from build123d import *

# Parameters (mm, degrees)
F0_W     = 122.6633450469
F0_H     = 164.7901384103
F0_W_2   = 102.3433450469
F0_H_2   = 144.4701384103
F1_DEPTH = 72.898
F2_R     = 8.301996535
F3_DEPTH = 244.094
F4_W     = 10.16
F4_H     = 88.5901384103
F5_DEPTH = 29.718


with BuildPart() as f1:
    # F0 (on Top) → F1 (new body)
    with BuildSketch(Plane.XY):
        with Locations((-22.7750174733, 0)):
            Rectangle(F0_W, F0_H)
        with Locations((-22.7750174733, 0)):
            Rectangle(F0_W_2, F0_H_2, mode=Mode.SUBTRACT)
    extrude(amount=F1_DEPTH)

    # F2 (on face) → F3 (cut)
    with BuildSketch(Plane(origin=(0, 82.3950692052, 0), x_dir=(-1, 0, 0), z_dir=(0, 1, 0))):
        with Locations((22.7750174733, 36.449)):
            Circle(F2_R)
    extrude(amount=-F3_DEPTH, mode=Mode.SUBTRACT)

    # F4 (on face) → F5 (cut)
    with BuildSketch(Plane.XY.offset(72.898)):
        with Locations((33.4766550502, 0)):
            Rectangle(F4_W, F4_H)
        with Locations((-79.0266899967, 0)):
            Rectangle(F4_W, F4_H)
    extrude(amount=-F5_DEPTH, mode=Mode.SUBTRACT)


solid = f1.part
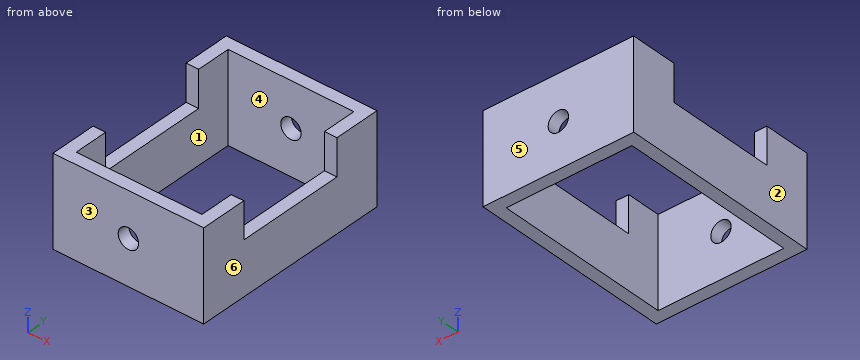
Input: part model. Units: mm. Frame: model coordinates. Face numbers are marked on the shaded views. A direction names the side the tool comes from. Coordinates: 2 decimals unless noted, no trailing zeros. Loops run counter-clockwise (first coordinate to the right, second up) from the corner with the lowest first, then second, coordinate; pieces in that order, holes last.
(1) Section D-D on z = 24.5. Return the cut outline in (x, y), then the cut area to 3 significant figures.
(2) Section B-B on x = 8. Return the cut outline in (y, z), then the cut area to 3 significant figures.
(3) Set-up query: the marked faces 1 and 2. Return all of +Z, -Z, +X, -X, +Y, -Y with unobstructed straight access to the full face (end or side cutting, diameter ignored); none if empty.
(4) Material intervals for probe 1 along X at (y, z) = (19, 43); probe 2 along Y at (x, z) = (-29.5, 24), sorted ascending.
(5) Section A-A on z = 54. Return the cut outline in (x, y), then the cut area to 3 significant figures.
(6) First-contact query: pin 1 Ø5 at (x, y) = (33.5, -4) entering from +Z; pin 2 Ø21.5 at (x, z) = (-22.78, 36.45) entering from -Y. Flat tips, straight axial feed; report the tip coordinate or a pass-through.
(7) Section C-C on y = -20. Return the cut outline in (x, z).
(8) Pull-direction query (Y, two-part tool) for the marked faces 3, 4, 5 and 6; classes: released by +Y, released by -Y, zero draft, split by the parting line, or undercut.
Data:
1. outline: (-84.11, -82.4) - (38.56, -82.4) - (38.56, 82.4) - (-84.11, 82.4) - close; hole (-73.95, -72.24) - (28.4, -72.24) - (28.4, 72.24) - (-73.95, 72.24) - close
1. area: 5,430 mm2
2. outline: (-82.4, 0) - (-72.24, 0) - (-72.24, 72.9) - (-82.4, 72.9) - close; (72.24, 0) - (82.4, 0) - (82.4, 72.9) - (72.24, 72.9) - close
2. area: 1,480 mm2
3. face 1: +Z, -Z
3. face 2: +Z, -Z, -X, +Y, -Y
4. probe 1: x = -84.11 to -73.95, 28.4 to 38.56
4. probe 2: y = -82.4 to -72.24, 72.24 to 82.4
5. outline: (-84.11, -82.4) - (38.56, -82.4) - (38.56, -44.3) - (28.4, -44.3) - (28.4, -72.24) - (-73.95, -72.24) - (-73.95, -44.3) - (-84.11, -44.3) - close; (-84.11, 44.3) - (-73.95, 44.3) - (-73.95, 72.24) - (28.4, 72.24) - (28.4, 44.3) - (38.56, 44.3) - (38.56, 82.4) - (-84.11, 82.4) - close
5. area: 3,630 mm2
6. pin 1: stops at z = 43.18
6. pin 2: stops at y = -82.4
7. outline: (-84.11, 0) - (-73.95, 0) - (-73.95, 43.18) - (-84.11, 43.18) - close; (28.4, 0) - (38.56, 0) - (38.56, 43.18) - (28.4, 43.18) - close
8. face 3: released by -Y
8. face 4: undercut
8. face 5: released by +Y
8. face 6: zero draft
